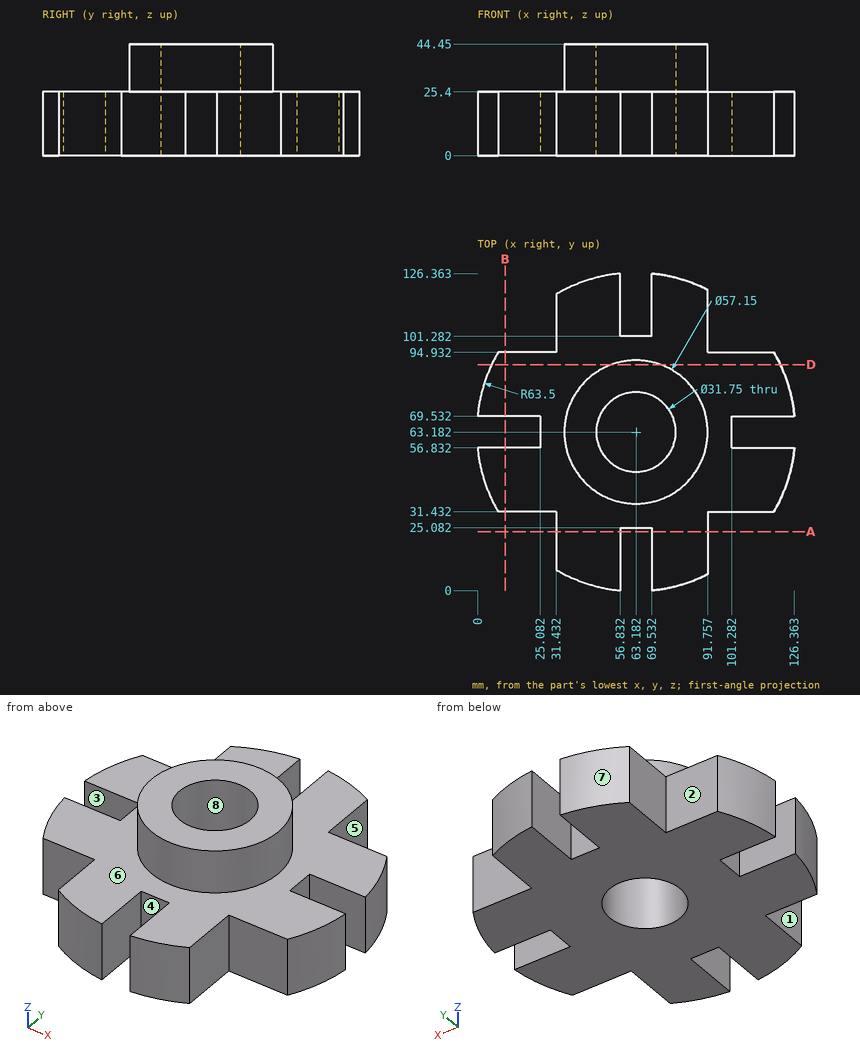
Design review of the part shown in the three views and the two pictorial views. Dimensions are in mm from the part's minimum x, y and z. A direction names the side the tool comes from. Coordinates: 2 decimals unless noted, no trailing zeros. Loops run counter-clockwise (first coordinate to the right, second up) from the corner with the lowest first, then second, coordinate; pieces in that order, holes last.
Q1. We need section D-D on y = 90. State the section outline as (x, z) points, and give its area (3 significant figures).
Reported:
outline: (5.62, 0) - (120.74, 0) - (120.74, 25.4) - (73.05, 25.4) - (73.05, 44.45) - (53.32, 44.45) - (53.32, 25.4) - (5.62, 25.4) - close
area: 3,300 mm2
Q2. We need section A-A on y = 23.5. State the section outline as (x, z) points.
Reported:
outline: (31.43, 0) - (56.83, 0) - (56.83, 25.4) - (31.43, 25.4) - close; (69.53, 0) - (91.76, 0) - (91.76, 25.4) - (69.53, 25.4) - close
Q3. To check wall thickness, follow line 1 (X direction, y = 16, z = 8); line 2 (X direction, y = 64, z = 19.5) (1 decimal); line 3 (Y direction, x = 19, z = 4). State the ranges of each line that lie inside material, in increasing order.
Reported:
line 1: x = 31.43 to 56.83, 69.53 to 91.76
line 2: x = 25.1 to 47.3, 79 to 101.3
line 3: y = 31.43 to 56.83, 69.53 to 94.93
Q4. Tool access review of the marked faces 1, 2, 3, 4 and 5: name each direction out of +Z, -Z, +X, -X, +Y, -Y from which nothing blocks a thin tool from reaching the whole face with its end or side.
Reported:
face 1: +Z, -Z, -X, -Y
face 2: +Z, -Z, -X, +Y
face 3: +Z, -Z, -X
face 4: +Z, -Z, -Y
face 5: +Z, -Z, +X, +Y
Q5. For pin 1 (1 mm diameter, centred on x = 46, z = 17.5, fed in from -Y); pin 2 (4 mm diameter, centred on x = 62.5, z = 9.5, fed in from +Y); pin 3 (12.5 mm diameter, centred on x = 7.5, z = 8.5, fed in from +Y); pin 4 (8 mm diameter, centred on x = 50.5, y = 72.5, fed in from +Z), all flat-tipped, find the tip position at first contact; note any pin that passes through.
Reported:
pin 1: stops at y = 1.91
pin 2: stops at y = 101.28
pin 3: stops at y = 94.93
pin 4: stops at z = 44.45
Q6. We need section B-B on x = 11. State the section outline as (y, z) points.
Reported:
outline: (31.43, 0) - (56.83, 0) - (56.83, 25.4) - (31.43, 25.4) - close; (69.53, 0) - (94.93, 0) - (94.93, 25.4) - (69.53, 25.4) - close
Q7. The part is to be moulded in two halves that separate along X. For the marked faces 6, 7 and 8, say which applies: +X half, -X half, draft (parallel to the pull), parting line (faces both ways), or undercut.
Reported:
face 6: draft
face 7: -X half
face 8: undercut
